```python
from build123d import *

# Parameters (mm, degrees)
F0_W     = 50
F0_H     = 35
F1_DEPTH = 13
F2_W     = 31
F2_H     = 20
F3_DEPTH = 20
F4_W     = 31
F4_H     = 7
F5_DEPTH = 27
F6_W     = 31
F6_H     = 2
F7_DEPTH = 13
F8_R     = 2.5
F9_DEPTH = 1.5


with BuildPart() as f1:
    # F0 (on Top) → F1 (new body)
    with BuildSketch(Plane.XY):
        Rectangle(F0_W, F0_H)
    extrude(amount=F1_DEPTH)

    # F2 (on face) → F3 (cut)
    with BuildSketch(Plane(origin=(-25, 0, 0), x_dir=(0, -1, 0), z_dir=(-1, 0, 0))):
        with Locations((0, 11)):
            Rectangle(F2_W, F2_H)
    extrude(amount=-F3_DEPTH, mode=Mode.SUBTRACT)

    # F4 (on face) → F5 (cut)
    with BuildSketch(Plane(origin=(-5, 0, 0), x_dir=(0, -1, 0), z_dir=(-1, 0, 0))):
        with Locations((0, 4.5)):
            Rectangle(F4_W, F4_H)
    extrude(amount=-F5_DEPTH, mode=Mode.SUBTRACT)

    # F6 (on face) → F7 (join)
    with BuildSketch(Plane(origin=(-5, 0, 0), x_dir=(0, -1, 0), z_dir=(-1, 0, 0))):
        with Locations((0, 9)):
            Rectangle(F6_W, F6_H)
    extrude(amount=F7_DEPTH)

    # F8 (on face) → F9 (cut)
    with BuildSketch(Plane.XY.offset(10)):
        with Locations((-12.5, 0)):
            Circle(F8_R)
    extrude(amount=-F9_DEPTH, mode=Mode.SUBTRACT)


solid = f1.part
```
Check sheet for the modelled part. Datum: model origin and axes. Units: mm. A direction names the side the tool comes from. Coordinates: 2 decimals unless noted, no trailing zeros. Write each loop counter-clockwise with the first axis right and the second up, starting at its lowest first coordinate (ties: lowest second). Pieces come first, ordered by that corner, then holes. Notation, with made-up numbers: M -6,35.5 L 14,35.5 A9 ccw 14,42.5 Z; hole C 21.5,-8 d11. An arc over 180 degrees is marked long. Write item = value, one per line. Start each with the question number.
1. Sectioned sample at D-D (x = 20.5). Record the cut outline in (y, z), then the cut area to 3 significant figures.
2. Sectioned sample at A-A (x = -12.5). Record the cut outline in (y, z).
3. Go/stop test with flat-tipped pins: pin 1 (3 mm diameter, centred on y = 1.5, z = 9, fed in from -X); pin 2 (6.5 mm diameter, centred on x = -11, y = 5.5, fed in from +Z); pin 3 (15.5 mm diameter, centred on x = -6.5, y = 6, fed in from -Z). Record where each tip stops, or that it passes through.
4. Sectioned sample at C-C (y = 0). Record the cut outline in (x, z), then the cut area to 4 significant figures.
5. Thickness scan on probe 1 along Y at (x, z) = (-18.5, 6.25); probe 2 along Z at (x, y) = (15, -9); probe 3 along Y at (x, z) = (-12.5, 9.6). Record the ranges inside material, lowest first.
6. Mould release check, pull along Y, two halves, no side actions. Record for faces 6 (the flat face through (-18, 0, 9)), 7 (the flat face through (-9, 0, 10)), 8 (the flat face through (0, -17.5, 6)), 9 (the flat face through (0, 17.5, 6)): pulls with the +Y half, pulls with the -Y half, needs draft (parallel to the pull), parting line crosses it, or undercut.
7. Sectioned sample at B-B (z = 3). Record the cut outline in (x, y), then the cut area to 3 significant figures.
8. Tool access check on faces 1 (the flat face through (-5, 0, 12)), 2 (the cylindrical face through (-15, 0, 9)), 3 (the flat face through (25, 0, 6)), 4 (the flat face through (-25, -4, 0.7)), 5 (the flat face through (-2, 0, 1)). Record the directions out of +Z, -Z, +X, -X, +Y, -Y that give a thin tool (end or side, any length) a straight path to the whole face; none if there is none.
The answers:
q1.outline = M -17.5,0 L 17.5,0 L 17.5,13 L -17.5,13 Z; hole M -15.5,1 L 15.5,1 L 15.5,8 L -15.5,8 Z
q1.area = 238 mm²
q2.outline = M -17.5,0 L 17.5,0 L 17.5,13 L 15.5,13 L 15.5,10 L 2.5,10 L 2.5,8.5 L -2.5,8.5 L -2.5,10 L -15.5,10 L -15.5,13 L -17.5,13 Z; hole M -15.5,1 L 15.5,1 L 15.5,8 L -15.5,8 Z
q3.pin_1 = -18
q3.pin_2 = 10
q3.pin_3 = 0
q4.outline = M -25,0 L 25,0 L 25,13 L -5,13 L -5,10 L -10,10 L -10,8.5 L -15,8.5 L -15,10 L -18,10 L -18,8 L 22,8 L 22,1 L -25,1 Z
q4.area = 239.5 mm²
q5.probe_1 = -17.5 to -15.5, 15.5 to 17.5
q5.probe_2 = 0 to 1, 8 to 13
q5.probe_3 = -17.5 to -2.5, 2.5 to 17.5
q6.face_6 = undercut
q6.face_7 = undercut
q6.face_8 = pulls with the -Y half
q6.face_9 = pulls with the +Y half
q7.outline = M -25,-17.5 L 25,-17.5 L 25,17.5 L -25,17.5 L -25,15.5 L 22,15.5 L 22,-15.5 L -25,-15.5 Z
q7.area = 293 mm²
q8.face_1 = +Z, -X
q8.face_2 = +Z
q8.face_3 = +Z, -Z, +X, +Y, -Y
q8.face_4 = +Z, -Z, -X, +Y, -Y
q8.face_5 = -X
